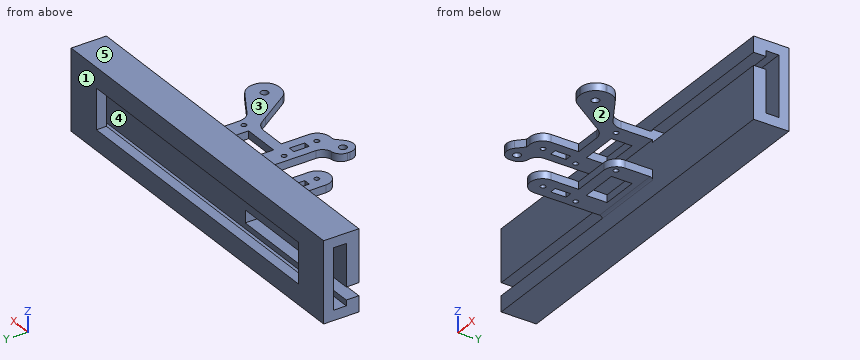
from build123d import *

# Parameters (mm, degrees)
SKETCH1_W            = 150
SKETCH1_H            = 32
BOSS_EXTRUDE1_DEPTH  = 5
SKETCH2_W            = 150
SKETCH2_H            = 4
BOSS_EXTRUDE2_DEPTH  = 9
SKETCH4_W            = 4
SKETCH4_H            = 4
BOSS_EXTRUDE3_DEPTH  = 150
SKETCH5_W            = 60
SKETCH5_H            = 5
CUT_EXTRUDE1_DEPTH   = 6
BOSS_EXTRUDE4_REACH  = 154.552
SKETCH6_W            = 15
SKETCH6_H            = 4
SKETCH7_W            = 60
SKETCH7_H            = 5
CUT_EXTRUDE2_DEPTH   = 6
SKETCH8_W            = 30
SKETCH8_H            = 3
BOSS_EXTRUDE5_DEPTH  = 16
SKETCH9_R            = 1
CUT_EXTRUDE3_DEPTH   = 153.867794188
SKETCH11_W           = 10
SKETCH11_H           = 3
BOSS_EXTRUDE7_DEPTH  = 16
SKETCH12_R           = 1
CUT_EXTRUDE4_DEPTH   = 156.359462216
SKETCH13_W           = 20
SKETCH13_H           = 3
BOSS_EXTRUDE8_DEPTH  = 20
SKETCH14_W           = 10
SKETCH14_H           = 3
BOSS_EXTRUDE9_DEPTH  = 4
SKETCH15_W           = 7
SKETCH15_H           = 3
BOSS_EXTRUDE10_DEPTH = 5
SKETCH16_R           = 1.5
CUT_EXTRUDE5_DEPTH   = 157.232399009
CUT_EXTRUDE6_DEPTH   = 5
CUT_EXTRUDE7_DEPTH   = 5
BOSS_EXTRUDE11_DEPTH = 3
CUT_EXTRUDE8_DEPTH   = 3
SKETCH21_W           = 14.847248178
SKETCH21_H           = 8.269274671
CUT_EXTRUDE9_DEPTH   = 157.232399009
FILLET3_R            = 6
FILLET4_R            = 4
FILLET5_R            = 5
FILLET6_R            = 5
SKETCH22_W           = 2.686432883
SKETCH22_H           = 6.135326584
CUT_EXTRUDE10_DEPTH  = 157.232399009
FILLET7_R            = 6
FILLET8_R            = 6
FILLET9_R            = 4
FILLET10_R           = 1
FILLET11_R           = 1


with BuildPart() as part:
    # Sketch1 → Boss-Extrude1 (new body)
    with BuildSketch(Plane(origin=(0, 0, 0), x_dir=(1, 0, 0), z_dir=(0, 1, 0))):
        with Locations((75, -16)):
            Rectangle(SKETCH1_W, SKETCH1_H)
    extrude(amount=BOSS_EXTRUDE1_DEPTH)

    # Sketch2 → Boss-Extrude2 (add)
    with BuildSketch(Plane(origin=(0, 5, 0), x_dir=(1, 0, 0), z_dir=(0, 1, 0))):
        with Locations((75, -30)):
            Rectangle(SKETCH2_W, SKETCH2_H)
        with Locations((75, -2)):
            Rectangle(SKETCH2_W, SKETCH2_H)
    extrude(amount=BOSS_EXTRUDE2_DEPTH)

    # Sketch4 → Boss-Extrude3 (add)
    with BuildSketch(Plane.ZY):
        with Locations((6, 12)):
            Rectangle(SKETCH4_W, SKETCH4_H)
        with Locations((26, 12)):
            Rectangle(SKETCH4_W, SKETCH4_H)
    extrude(amount=-BOSS_EXTRUDE3_DEPTH)

    # Sketch5 → Cut-Extrude1 (cut)
    with BuildSketch(Plane(origin=(0, 0, 0), x_dir=(-1, 0, 0), z_dir=(0, -1, 0))):
        with Locations((-120, -23.25)):
            Rectangle(SKETCH5_W, SKETCH5_H)
    extrude(amount=-CUT_EXTRUDE1_DEPTH, mode=Mode.SUBTRACT)

    # Sketch6 → Boss-Extrude4 (add, up to next)
    with BuildSketch(Plane(origin=(0, 0, 24), x_dir=(-1, 0, 0), z_dir=(0, 0, -1)), mode=Mode.PRIVATE) as boss_extrude4_sk1:
        with Locations((-142.5, 12)):
            Rectangle(SKETCH6_W, SKETCH6_H)
    boss_extrude4_tool1 = extrude(boss_extrude4_sk1.sketch, amount=BOSS_EXTRUDE4_REACH, mode=Mode.PRIVATE) - part.part
    # Sketch6 → Boss-Extrude4 (add, up to next)
    with BuildSketch(Plane(origin=(0, 0, 24), x_dir=(-1, 0, 0), z_dir=(0, 0, -1)), mode=Mode.PRIVATE) as boss_extrude4_sk2:
        with Locations((-7.5, 12)):
            Rectangle(SKETCH6_W, SKETCH6_H)
    boss_extrude4_tool2 = extrude(boss_extrude4_sk2.sketch, amount=BOSS_EXTRUDE4_REACH, mode=Mode.PRIVATE) - part.part
    add(boss_extrude4_tool1.solids().sort_by_distance((142.5, 12, 24))[0])
    add(boss_extrude4_tool2.solids().sort_by_distance((7.5, 12, 24))[0])

    # Sketch7 → Cut-Extrude2 (cut)
    with BuildSketch(Plane(origin=(0, 0, 0), x_dir=(-1, 0, 0), z_dir=(0, -1, 0))):
        with Locations((-30, -8.75)):
            Rectangle(SKETCH7_W, SKETCH7_H)
    extrude(amount=-CUT_EXTRUDE2_DEPTH, mode=Mode.SUBTRACT)

    # Sketch8 → Boss-Extrude5 (add)
    with BuildSketch(Plane.XZ):
        with Locations((75, 23.25)):
            Rectangle(SKETCH8_W, SKETCH8_H)
        with Locations((75, 8.75)):
            Rectangle(SKETCH8_W, SKETCH8_H)
    extrude(amount=BOSS_EXTRUDE5_DEPTH)

    # Sketch9 → Cut-Extrude3 (cut, through all)
    with BuildSketch(Plane(origin=(0, 0, 7.25), x_dir=(-1, 0, 0), z_dir=(0, 0, -1))):
        with Locations((-63, -12.5)):
            Circle(SKETCH9_R)
        with Locations((-87, -12.5)):
            Circle(SKETCH9_R)
    extrude(amount=-CUT_EXTRUDE3_DEPTH, mode=Mode.SUBTRACT)

    # Sketch11 → Boss-Extrude7 (add)
    with BuildSketch(Plane(origin=(0, -16, 0), x_dir=(-1, 0, 0), z_dir=(0, -1, 0))):
        with Locations((-65, -8.75)):
            Rectangle(SKETCH11_W, SKETCH11_H)
        with Locations((-65, -23.25)):
            Rectangle(SKETCH11_W, SKETCH11_H)
    extrude(amount=BOSS_EXTRUDE7_DEPTH)

    # Sketch12 → Cut-Extrude4 (cut, through all)
    with BuildSketch(Plane.XY.offset(24.75)):
        with Locations((65, -26.8)):
            Circle(SKETCH12_R)
    extrude(amount=-CUT_EXTRUDE4_DEPTH, mode=Mode.SUBTRACT)

    # Sketch13 → Boss-Extrude8 (add)
    with BuildSketch(Plane(origin=(0, -16, 0), x_dir=(-1, 0, 0), z_dir=(0, -1, 0))):
        with Locations((-97, -23.25)):
            Rectangle(SKETCH13_W, SKETCH13_H)
    extrude(amount=BOSS_EXTRUDE8_DEPTH)

    # Sketch14 → Boss-Extrude9 (add)
    with BuildSketch(Plane(origin=(0, -32, 0), x_dir=(-1, 0, 0), z_dir=(0, -1, 0))):
        with Locations((-58, -23.25)):
            Rectangle(SKETCH14_W, SKETCH14_H)
    extrude(amount=BOSS_EXTRUDE9_DEPTH)

    # Sketch15 → Boss-Extrude10 (add)
    with BuildSketch(Plane(origin=(0, -32, 0), x_dir=(1, 0, 0), z_dir=(0, 1, 0))):
        with Locations((56.5, -23.25)):
            Rectangle(SKETCH15_W, SKETCH15_H)
    extrude(amount=BOSS_EXTRUDE10_DEPTH)

    # Sketch16 → Cut-Extrude5 (cut, through all)
    with BuildSketch(Plane.XY.offset(24.75)):
        with Locations((56.830024482, -31.707497886)):
            Circle(SKETCH16_R)
        with Locations((100.640738332, -29.851736065)):
            Circle(SKETCH16_R)
    extrude(amount=-CUT_EXTRUDE5_DEPTH, mode=Mode.SUBTRACT)

    # Sketch17 → Cut-Extrude6 (cut)
    with BuildSketch(Plane.XY.offset(24.75)):
        Polygon((97, -36), (87, -21.056914339), (87, -36), align=None)
    extrude(amount=-CUT_EXTRUDE6_DEPTH, mode=Mode.SUBTRACT)

    # Sketch18 → Cut-Extrude7 (cut)
    with BuildSketch(Plane.XY.offset(24.75)):
        Polygon((107, -26), (90, -16), (107, -16), align=None)
    extrude(amount=-CUT_EXTRUDE7_DEPTH, mode=Mode.SUBTRACT)

    # Sketch19 → Boss-Extrude11 (add)
    with BuildSketch(Plane.XY.offset(24.75)):
        Polygon((87, -21.056914339), (83.615883457, -16), (87, -16), align=None)
    extrude(amount=-BOSS_EXTRUDE11_DEPTH)

    # Sketch20 → Cut-Extrude8 (cut)
    with BuildSketch(Plane.XY.offset(24.75)):
        Polygon((58.822210862, -36), (63, -32), (63, -36), align=None)
    extrude(amount=-CUT_EXTRUDE8_DEPTH, mode=Mode.SUBTRACT)

    # Sketch21 → Cut-Extrude9 (cut, through all)
    with BuildSketch(Plane(origin=(0, 0, 7.25), x_dir=(-1, 0, 0), z_dir=(0, 0, -1))):
        with Locations((-75.571857051, -7.603356602)):
            Rectangle(SKETCH21_W, SKETCH21_H)
    extrude(amount=-CUT_EXTRUDE9_DEPTH, mode=Mode.SUBTRACT)

    # Fillet3
    fillet3_edges = [part.edges().sort_by_distance(p)[0] for p in [
        (107, -36, 23.25),
        (97, -36, 23.25),
        (107, -26, 23.25),
    ]]
    fillet(fillet3_edges, radius=FILLET3_R)

    # Fillet4
    fillet4_edges = [part.edges().sort_by_distance(p)[0] for p in [
        (53, -36, 23.25),
        (53, -27, 23.25),
        (58.822210862, -36, 23.25),
    ]]
    fillet(fillet4_edges, radius=FILLET4_R)

    # Fillet5
    fillet5_edges = [part.edges().sort_by_distance(p)[0] for p in [
        (90, -16, 8.75),
        (70, -32, 8.75),
        (60, -32, 8.75),
    ]]
    fillet(fillet5_edges, radius=FILLET5_R - 0.0001)  # a hair under: the kernel refuses the full size

    # Fillet6
    fillet6_edges = [part.edges().sort_by_distance(p)[0] for p in [
        (70, -32, 23.25),
    ]]
    fillet(fillet6_edges, radius=FILLET6_R)

    # Sketch22 → Cut-Extrude10 (cut, through all)
    with BuildSketch(Plane(origin=(0, 0, 7.25), x_dir=(-1, 0, 0), z_dir=(0, 0, -1))):
        with Locations((-64.85928039, -19.744776936)):
            Rectangle(SKETCH22_W, SKETCH22_H)
    extrude(amount=-CUT_EXTRUDE10_DEPTH, mode=Mode.SUBTRACT)

    # Fillet7
    fillet7_edges = [part.edges().sort_by_distance(p)[0] for p in [
        (90, -16, 23.25),
    ]]
    fillet(fillet7_edges, radius=FILLET7_R)

    # Fillet8
    fillet8_edges = [part.edges().sort_by_distance(p)[0] for p in [
        (83.615883457, -16, 23.25),
    ]]
    fillet(fillet8_edges, radius=FILLET8_R)

    # Fillet9
    fillet9_edges = [part.edges().sort_by_distance(p)[0] for p in [
        (60, -27, 23.25),
    ]]
    fillet(fillet9_edges, radius=FILLET9_R)

    # Fillet10
    fillet10_edges = [part.edges().sort_by_distance(p)[0] for p in [
        (75, 0, 7.25),
    ]]
    fillet(fillet10_edges, radius=FILLET10_R)

    # Fillet11
    fillet11_edges = [part.edges().sort_by_distance(p)[0] for p in [
        (75, 0, 24.75),
    ]]
    fillet(fillet11_edges, radius=FILLET11_R)


solid = part.part
Input: part model. Units: mm. Frame: model coordinates. Face numbers are marked on the shaded views. A direction names the side the tool comes from. Coordinates: 2 decimals unless noted, no trailing zeros. Loops run counter-clockwise (first coordinate to the right, second up) from the corner with the lowest first, then second, coordinate; pieces in that order, holes last.
Q1. Cut plane B-B (z = 18.5). Output: boundary loops of the cut face in (x, y).
Q2. Cut plane C-C (x = 71.5). Give the number of separate pieces and of enclosed holes in the cut face, then the cut area to 3 significant figures.
Q3. Contact query for flat-ended pins moving along their axis: pin 1 (1.5 mm diameter, centred on y = -8, z = 23, fed in from -X); pin 2 (2.5 mm diameter, centred on y = 0, z = 22.5, fed in from +X); pin 3 (2.5 mm diameter, centred on y = -21.5, z = 8.5, fed in from +X). Output: stop coordinate, or through.
Q4. Set-up query: the marked faces 4 and 5. Return all of +Z, -Z, +X, -X, +Y, -Y with unobstructed straight access to the full face (end or side cutting, diameter ignored); none if empty.
Q5. Material intervals for line 1 (Z direction, x = 80, y = 6); line 2 (Y direction, x = 13, z = 15); line 3 (Z direction, x = 111, y = 4), sorted ascending.
Q6. Draft query along Z for the marked faces 1, 2 and 3. Return one class per face: +Z half, -Z half, draft (parallel to the pull), parting line (faces both ways), or undercut.
Q7. Cut plane D-D (x = 120.5). Output: boundary loops of the cut face in (y, z), then the cut area to 3 significant figures.
Q8. Cut plane A-A (y = -7). Output: boundary loops of the cut face in (x, z), then the cut area to 3 significant figures.
Working result:
1. outline: (0, 0) - (150, 0) - (150, 5) - (0, 5) - close; (0, 10) - (15, 10) - (15, 14) - (0, 14) - close; (135, 10) - (150, 10) - (150, 14) - (135, 14) - close
2. separate pieces: 3
2. enclosed holes: 0
2. area: 311 mm2
3. pin 1: stops at x = 60
3. pin 2: stops at x = 90
3. pin 3: stops at x = 70
4. face 4: +X, -X
4. face 5: +Z, +X, -X, +Y, -Y
5. line 1: z = 0 to 4, 28 to 32
5. line 2: y = 0 to 5, 10 to 14
5. line 3: z = 0 to 20.75, 25.75 to 32
6. face 1: draft
6. face 2: undercut
6. face 3: +Z half
7. outline: (0, 0) - (14, 0) - (14, 8) - (10, 8) - (10, 4) - (5, 4) - (5, 20.75) - (0, 20.75) - close; (0, 25.75) - (5, 25.75) - (5, 28) - (10, 28) - (10, 24) - (14, 24) - (14, 32) - (0, 32) - close
7. area: 239 mm2
8. outline: (60, 7.25) - (68.15, 7.25) - (68.15, 10.25) - (60, 10.25) - close; (60, 21.75) - (68.15, 21.75) - (68.15, 24.75) - (60, 24.75) - close; (83, 7.25) - (90, 7.25) - (90, 10.25) - (83, 10.25) - close; (83, 21.75) - (90, 21.75) - (90, 24.75) - (83, 24.75) - close
8. area: 90.9 mm2
